The model under review builds one solid part; all positions refer to its coordinate system, in mm. Face numbers are marked on the shaded views. A direction names the side the tool comes from. Round coordinates to 2 decimals unless told otherwise and drop trailing zeros. Loops run counter-clockwise (first coordinate to the right, second up) from the corner with the lowest first, then second, coordinate; pieces in that order, holes last. Notation, with made-up numbers: (79.25, 36) -> (115.25, 36) arc R26 cw to (115.25, 50) -> close; hole circle Ø7 at (-1.75, -29). An arc over 180 degrees is marked (long way). Use a Markdown table: item, result. Add a question column.
1) Consider section A-A on x = 0. Give the boundary of the cut face in (y, z) (1 decimal).
2) Consider section D-D on y = 2.2. Give the boundary of the cut face in (x, z).
3) For the marked faces 4 and 5, list the 3-axis set-ups (+Z, -Z, +X, -X, +Y, -Y) from which the entire face can be reached by the end or side of a thin tool; tool diameter is ignored.
4) Insertion check: pin 1 (3 mm diameter, centred on x = 3.5, y = 0.5, fed in from +Z); pin 2 (1.5 mm diameter, centred on x = 5.5, y = 3.5, fed in from +Z); pin 3 (6 mm diameter, centred on x = -5.5, z = -3, fed in from -Y); pin 4 (8.5 mm diameter, centred on x = 0, z = 0, fed in from +Y) (3 decimals). Each pin has a flat end and moves straight along its axis. Give the tip position at first contact, or say it passes through.
5) Consider section B-B on y = 3.7. Give the boundary of the cut face in (x, z), plus the area to 3 significant figures.
6) Mouldability with a two-part tool opening along X and no side actions: class the marked faces 1, 2 and 3 as released by +X, released by -X, zero draft, split by the parting line, or undercut.
7) Wall thickness on probe 1 along X at (y, z) = (0.8, 0); probe 2 along Y at (x, z) = (6, 2.75) (3 decimals): over which ranges is each line inside the solid? List them lowest first.
8) Consider section C-C on z = -2.25. Give the boundary of the cut face in (x, y) (3 decimals), plus the area to 3 significant figures.
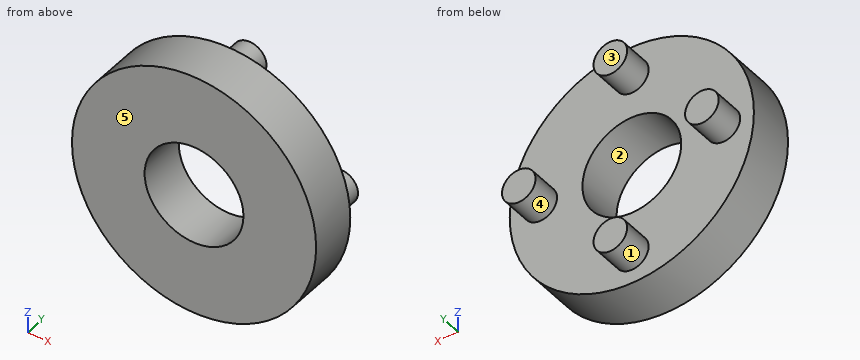
from build123d import *

# Parameters (mm, degrees)
SKETCH1_R           = 8
SKETCH1_R_2         = 3.2385
BOSS_EXTRUDE1_DEPTH = 3.175
SKETCH2_R           = 1.1
BOSS_EXTRUDE2_DEPTH = 2


with BuildPart() as part:
    # Sketch1 → Boss-Extrude1 (new body)
    with BuildSketch(Plane(origin=(0, 0, 0), x_dir=(1, 0, 0), z_dir=(0, 1, 0))):
        Circle(SKETCH1_R)
        Circle(SKETCH1_R_2, mode=Mode.SUBTRACT)
    extrude(amount=BOSS_EXTRUDE1_DEPTH)

    # Sketch2 → Boss-Extrude2 (add)
    with BuildSketch(Plane(origin=(0, 3.175, 0), x_dir=(1, 0, 0), z_dir=(0, 1, 0))):
        with Locations((0, 6)):
            Circle(SKETCH2_R)
        with Locations((6, 0)):
            Circle(SKETCH2_R)
        with Locations((0, -6)):
            Circle(SKETCH2_R)
        with Locations((-6, 0)):
            Circle(SKETCH2_R)
    extrude(amount=BOSS_EXTRUDE2_DEPTH)


solid = part.part
Result set:
| question | item | result |
|---|---|---|
| 1 | outline | (0, -8) -> (3.2, -8) -> (3.2, -7.1) -> (5.2, -7.1) -> (5.2, -4.9) -> (3.2, -4.9) -> (3.2, -3.2) -> (0, -3.2) -> close; (0, 3.2) -> (3.2, 3.2) -> (3.2, 4.9) -> (5.2, 4.9) -> (5.2, 7.1) -> (3.2, 7.1) -> (3.2, 8) -> (0, 8) -> close |
| 2 | outline | circle Ø16 at (0, 0); hole circle Ø6.48 at (0, 0) |
| 3 | face 4 | +Y |
| 3 | face 5 | +Z, -Z, +X, -X, -Y |
| 4 | pin 1 | z = 7.75 |
| 4 | pin 2 | z = 6.38 |
| 4 | pin 3 | y = 0 |
| 4 | pin 4 | y = 3.175 |
| 5 | outline | circle Ø2.2 at (-6, 0); circle Ø2.2 at (0, -6); circle Ø2.2 at (0, 6); circle Ø2.2 at (6, 0) |
| 5 | area | 15.2 mm2 |
| 6 | face 1 | split by the parting line |
| 6 | face 2 | undercut |
| 6 | face 3 | zero draft |
| 7 | probe 1 | -8 to -3.24, 3.24 to 8 |
| 7 | probe 2 | 0 to 3.175 |
| 8 | outline | (-7.677, 0) -> (-2.329, 0) -> (-2.329, 3.175) -> (-7.677, 3.175) -> close; (2.329, 0) -> (7.677, 0) -> (7.677, 3.175) -> (2.329, 3.175) -> close |
| 8 | area | 34.0 mm2 |
